Read the model definition and answer for the solid it produces. Units are mm, in the model's axes. Face numbers are marked on the shaded views. A direction names the side the tool comes from. Coordinates: 2 decimals unless noted, no trailing zeros. Write each loop counter-clockwise with the first axis right and the second up, starting at its lowest first coordinate (ties: lowest second). Pieces come first, ordered by that corner, then holes. Notation, with made-up numbers: (60, 85) - (106, 85) arc R20 cw to (106, 95) - close; hole circle Ø9 at (79, 65.5). An arc over 180 degrees is marked (long way). Return JSON: item names as keys, results as strings.
```python
from build123d import *
from build123d.topology import SkipClean

# Parameters (mm, degrees)
SKETCH1_R               = 2.625
BOSS_EXTRUDE1_DEPTH     = 18
SKETCH2_W               = 3.75
SKETCH2_H               = 40
BOSS_EXTRUDE2_DEPTH     = 15.5
CUT_EXTRUDE2_DEPTH      = 3.5
CUT_EXTRUDE2_DEPTH_BACK = 3.5
SKETCH4_W               = 26.185074211
SKETCH4_H               = 43.492971865
CUT_EXTRUDE3_DEPTH      = 3.75
CUT_EXTRUDE4_DEPTH      = 4
SKETCH6_R               = 4.5
CUT_EXTRUDE5_DEPTH      = 2


with BuildPart() as part:
    # Sketch1 → Boss-Extrude1 (new body)
    with BuildSketch(Plane(origin=(0, 0, 0), x_dir=(0, 0, -1), z_dir=(1, 0, 0))):
        with BuildLine():
            Line((0, 0), (5, 0))
            Line((5, 0), (5, 40))
            Line((5, 40), (0, 40))
            Line((0, 40), (-2.5, 40))
            Line((-2.5, 40), (-15.763202528, 42.911607583))
            ThreePointArc((-15.763202528, 42.911607583), (-22.576511621, 41.311816677), (-25.6, 35))
            Line((-25.6, 35), (-25.6, 20))
            ThreePointArc((-25.6, 20), (-24.659331675, 16.211336651), (-22.055809883, 13.302642588))
            Line((-22.055809883, 13.302642588), (-2.5, 0))
            Line((-2.5, 0), (0, 0))
        make_face()
        with Locations((-17.5, 35)):
            Circle(SKETCH1_R, mode=Mode.SUBTRACT)
        with Locations((-17.5, 20)):
            Circle(SKETCH1_R, mode=Mode.SUBTRACT)
    extrude(amount=BOSS_EXTRUDE1_DEPTH)

    # Sketch2 → Boss-Extrude2 (add)
    with BuildSketch(Plane.ZY):
        with Locations((-3.125, 20)):
            Rectangle(SKETCH2_W, SKETCH2_H)
    extrude(amount=BOSS_EXTRUDE2_DEPTH)

    # Sketch4 → Cut-Extrude2 (cut, two sides: drawn at the far end of the back side and taken through both)
    with BuildSketch(Plane(origin=(9, 0, 0), x_dir=(0, 0, -1), z_dir=(1, 0, 0)).offset(-CUT_EXTRUDE2_DEPTH_BACK)):
        with Locations((-19.842537105, 21.746485933)):
            Rectangle(SKETCH4_W, SKETCH4_H)
    extrude(amount=CUT_EXTRUDE2_DEPTH + CUT_EXTRUDE2_DEPTH_BACK, mode=Mode.SUBTRACT)

    # Sketch5 → Cut-Extrude3 (cut)
    with BuildSketch(Plane.XY.offset(-1.25)):
        with BuildLine():
            Line((-15.5, 23.302), (-15.5, 16.698))
            ThreePointArc((-15.5, 16.698), (-12.198, 20), (-15.5, 23.302))
        make_face()
    extrude(amount=-CUT_EXTRUDE3_DEPTH, mode=Mode.SUBTRACT)

    # Sketch3 → Cut-Extrude4 (cut)
    with BuildSketch(Plane(origin=(0, 0, 0), x_dir=(0, 0, -1), z_dir=(1, 0, 0))):
        Polygon((-12.881197846, 35), (-15.190598923, 39), (-19.809401077, 39), (-22.118802154, 35), (-19.809401077, 31), (-15.190598923, 31), align=None)
        Polygon((-12.881197846, 20), (-15.190598923, 24), (-19.809401077, 24), (-22.118802154, 20), (-19.809401077, 16), (-15.190598923, 16), align=None)
    extrude(amount=CUT_EXTRUDE4_DEPTH, mode=Mode.SUBTRACT)

    # Sketch6 → Cut-Extrude5 (cut)
    with BuildSketch(Plane(origin=(18, 0, 0), x_dir=(0, 0, -1), z_dir=(1, 0, 0))):
        with Locations((-17.5, 20)):
            Circle(SKETCH6_R)
        with Locations((-17.5, 35)):
            Circle(SKETCH6_R)
    extrude(amount=-CUT_EXTRUDE5_DEPTH, mode=Mode.SUBTRACT)

    # Mirror2: part across plane


with BuildPart() as part_1:
    with SkipClean():  # the faces are left unmerged after this step: merging them gives an invalid solid
        add(part.part)
        add(part.part.mirror(Plane(origin=(-15.5, 0, 0), x_dir=(0, 0, 1), z_dir=(1, 0, 0))))


solid = part_1.part
```
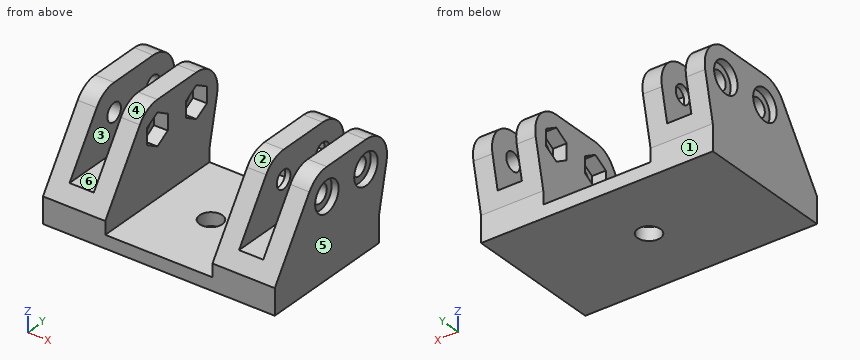
(1) A cutting plane is placed at C-C (y = 29.5). Determine the outline of the cut face in (x, z), and give its area (3 significant figures).
Answer:
{"outline": "(-49, -5) - (18, -5) - (18, 25.6) - (12.5, 25.6) - (12.5, 6.75) - (5.5, 6.75) - (5.5, 25.6) - (0, 25.6) - (0, -1.25) - (-31, -1.25) - (-31, 25.6) - (-36.5, 25.6) - (-36.5, 6.75) - (-43.5, 6.75) - (-43.5, 25.6) - (-49, 25.6) - close", "area": "954 mm²"}
(2) Flat-ended cylindrical pins translate along their axes: P1, Ø8, axis at y = 7, z = 15, coming from the +X side; P2, Ø2.5, axis at y = 18.5, z = 16.5, coming from the +X side; P3, Ø8, axis at x = 9.5, z = 6, coming from the +Y side; P4, Ø2.5, axis at y = 34.5, z = 18.5, coming from the +X side. Find the tip coordinate at first contact, or state that the pin passes through.
Answer:
{"P1": "x = 18", "P2": "x = 16", "P3": "y = 41.35", "P4": "through"}
(3) A cutting plane is placed at D-D (z = 9). Determine the outline of the cut face in (x, y).
Answer:
{"outline": "(-49, 4.42) - (-43.5, 4.42) - (-43.5, 41.43) - (-49, 41.43) - close; (-36.5, 4.42) - (-31, 4.42) - (-31, 41.43) - (-36.5, 41.43) - close; (0, 4.42) - (5.5, 4.42) - (5.5, 41.43) - (0, 41.43) - close; (12.5, 4.42) - (18, 4.42) - (18, 41.43) - (12.5, 41.43) - close"}
(4) Determine the mould class of the marked faces 4, 5 and 6 for opening direction X: +X half, -X half, draft (parallel to the pull), parting line (faces both ways), or undercut.
Answer:
{"face 4": "draft", "face 5": "+X half", "face 6": "undercut"}
(5) Which of the six approach directions +Z, -Z, +X, -X, +Y, -Y give full straight-line access (tool end or side, diameter ignored) to the marked faces 1, 2 and 3?
Answer:
{"face 1": "-Z, +X, -X, +Y", "face 2": "+Z, +X, -X, -Y", "face 3": "+Z, +Y, -Y"}
(6) A cutting plane is placed at A-A (z = 0.5). Determine the outline of the cut face in (x, y), and give its area (3 significant figures).
Answer:
{"outline": "(-49, 0) - (-31, 0) - (-31, 40) - (-49, 40) - close; (0, 0) - (18, 0) - (18, 40) - (0, 40) - close", "area": "1,440 mm²"}
(7) Straight lines are drawn through the part: line 1 (X direction, y = 34.5, z = 12); line 2 (X direction, y = 38, z = 15.5); line 3 (Y direction, x = 13.8, z = 17.5) (3 decimals). For each, find the intervals that lie inside material, in ascending order. Write a range as from..to.
Answer:
{"line 1": "-49..-43.5, -36.5..-31, 0..5.5, 12.5..18", "line 2": "-47..-43.5, -36.5..-35, 4..5.5, 12.5..16", "line 3": "10.204..17.375, 22.625..32.375, 37.625..43.1"}
(8) A cutting plane is placed at B-B (x = -15.5). Determine the outline of the cut face in (y, z).
Answer:
{"outline": "(0, -5) - (16.7, -5) - (16.7, -1.25) - (0, -1.25) - close; (23.3, -5) - (40, -5) - (40, -1.25) - (23.3, -1.25) - close"}
